Design review of the part shown in the three views and the two pictorial views. Dimensions are in mm from the part's minimum x, y and z. A direction names the side the tool comes from. Give positions to 0.01 mm unless a question says otherwise; leave off trailing zeros. Loops run counter-clockwise (first coordinate to the right, second up) from the corner with the lowest first, then second, coordinate; pieces in that order, holes last.
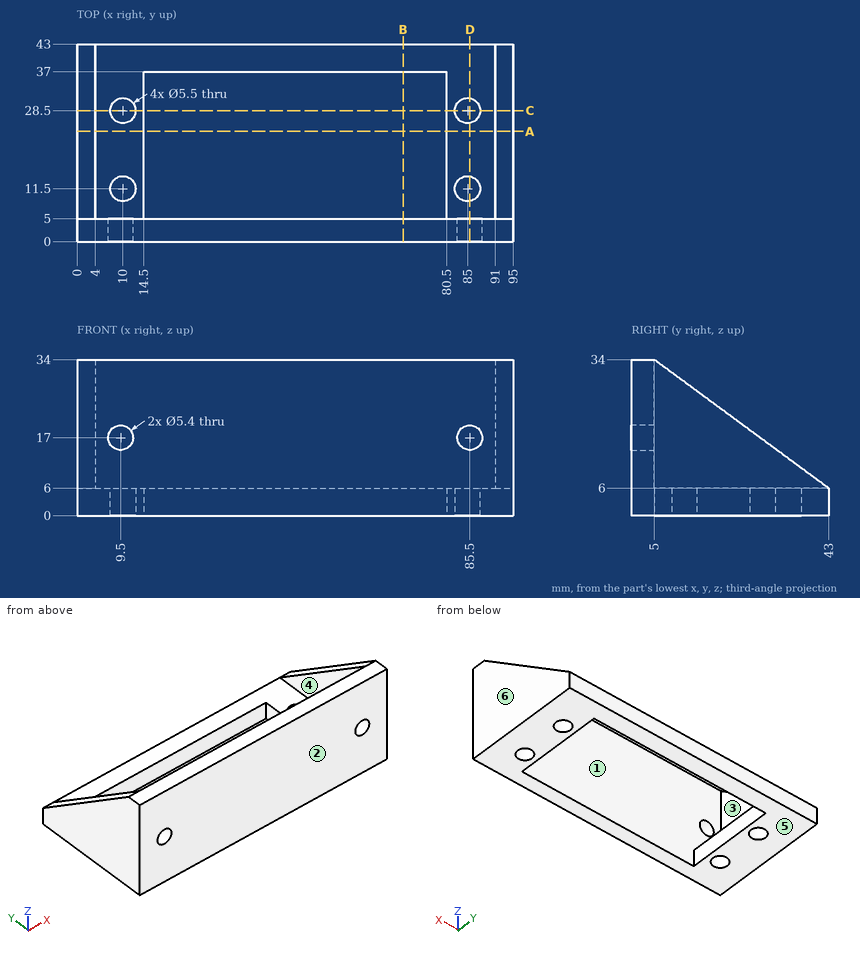
Q1. Consider section B-B on x = 71. Give the boundary of the cut face in (y, z), plus the area to 3 significant figures.
Answers:
outline: (0, 0) - (5, 0) - (5, 34) - (0, 34) - close; (37, 0) - (43, 0) - (43, 6) - (37, 6) - close
area: 206 mm2
Q2. For pin 1 Ø6 at (x, z) = (85.5, 17) entering from +Y; pin 2 Ø3 at (x, y) = (14.5, 28) entering from +Z, all flat-tipped, find the tip position at first contact; note any pin that passes through.
Answers:
pin 1: stops at y = 5
pin 2: stops at z = 6
Q3. Machinability: for the marked faces 1, 2 and 3, which of the approach directions +Z, -Z, +X, -X, +Y, -Y give a long, thin tool a straight path to every point of the face, cutting with its end or side? Answer none if there is none.
Answers:
face 1: +Z
face 2: +Z, -Z, +X, -X, -Y
face 3: +Z, +Y
Q4. Consider section D-D on x = 85.5. Give the boundary of the cut face in (y, z), plus the area to 3 significant figures.
Answers:
outline: (0, 0) - (8.8, 0) - (8.8, 6) - (5, 6) - (5, 14.3) - (0, 14.3) - close; (0, 19.7) - (5, 19.7) - (5, 34) - (0, 34) - close; (14.2, 0) - (25.8, 0) - (25.8, 6) - (14.2, 6) - close; (31.2, 0) - (43, 0) - (43, 6) - (31.2, 6) - close
area: 306 mm2
Q5. Consider section C-C on y = 28.5. Give the boundary of the cut face in (x, z).
Answers:
outline: (0, 0) - (7.25, 0) - (7.25, 6) - (4, 6) - (4, 16.68) - (0, 16.68) - close; (12.75, 0) - (14.5, 0) - (14.5, 6) - (12.75, 6) - close; (80.5, 0) - (82.25, 0) - (82.25, 6) - (80.5, 6) - close; (87.75, 0) - (95, 0) - (95, 16.68) - (91, 16.68) - (91, 6) - (87.75, 6) - close
Q6. For probe 1 along Y at (x, z) = (85, 1.6); probe 2 along X at (y, z) = (2.7, 17); probe 3 along X at (y, z) = (21.5, 15), list the stretches that pass through material, from the lowest coordinate up.
Answers:
probe 1: y = 0 to 8.75, 14.25 to 25.75, 31.25 to 43
probe 2: x = 0 to 6.8, 12.2 to 82.8, 88.2 to 95
probe 3: x = 0 to 4, 91 to 95
Q7. Mouldability with a two-part tool opening along X and no side actions: class the marked faces 4, 5 and 6 as +X half, -X half, draft (parallel to the pull), parting line (faces both ways), or undercut.
Answers:
face 4: undercut
face 5: draft
face 6: +X half
Q8. Consider section A-A on y = 24. Give the boundary of the cut face in (x, z), plus the area to 3 significant figures.
Answers:
outline: (0, 0) - (14.5, 0) - (14.5, 6) - (4, 6) - (4, 20) - (0, 20) - close; (80.5, 0) - (95, 0) - (95, 20) - (91, 20) - (91, 6) - (80.5, 6) - close
area: 286 mm2
